Source: CAD feature listing. Evaluate the final solid. Frame: model axes, mm. A direction names the side the tool comes from. Round coordinates to 2 decimals unless told otherwise and drop trailing zeros. Order: outer loops, then holes, each group sorted by start corner. A loop starts at its lowest first (then second) coordinate and runs counter-clockwise, first axis right, second up. Notation, with made-up numbers: M 53,-7 L 66,-7 A14 cw 66,5 Z; hole C 20.25,48.25 d3. An arc over 180 degrees is marked long. Answer as CSV lines item,"result". Start each with the question number.
Item 1: Section query A-A on y = 9.75. Return the cut outline in (x, z).
Item 2: First-contact query: P1, Ø5.5, axis at x = 31, z = -31, coming from the +Y side; P2, Ø1.5, axis at x = 12.5, z = -29.5, coming from the +Y side. Flat tips, straight axial feed; report the tip coordinate or a pass-through.
Item 3: Set-up query: faces 4 (the face through (47.926, 8.378, -56.352)), 5 (the face through (12, 8.1, -30)), 6 (the face through (27, 6.4, -30)). Return all of +Z, -Z, +X, -X, +Y, -Y with unobstructed straight access to the full face (end or side cutting, diameter ignored); none if empty.
Item 4: Pull-direction query (Y, two-part tool) for faces 1 (the face through (9.62, 11, -30)), 2 (the face through (42.76, 15.983, -29.58)), 3 (the face through (4.14, 8.378, -56.983)); classes: +Y half, -Y half, draft (parallel to the pull), parting line (faces both ways), or undercut.
Item 5: Section query B-B on z = -5. State how many separate pieces and enclosed holes the cut face has, plus the area to 3 significant figures.
Item 6: Section query D-D on y = 3.5. Return the cut outline in (x, z), plus the area to 3 significant figures.
Item 7: Section query C-C on x = 49.4. Return the cut outline in (y, z) (3 decimals).
Item 8: Line query: line 1 (X direction, y = 7, z = -55); line 2 (X direction, y = 9, z = -24); line 3 (Z direction, x = 4.4, y = 4). Output: solid intervals per line, ascending. Write a range as [from, to].
from build123d import *

# Parameters (mm, degrees)
BOSS_EXTRUDE1_DEPTH             = 60
F_4_0MM_DOWEL_HOLE1_D           = 4
F_4_0MM_DOWEL_HOLE1_CSINK_D     = 4.05
F_4_0MM_DOWEL_HOLE1_CSINK_ANGLE = 90


with BuildPart() as part:
    # Sketch2 → Boss-Extrude1 (new body)
    with BuildSketch(Plane.XY):
        Polygon((36.38, 6.4), (26.9, 6.4), (26.9, 0), (53.8, 0), (53.8, 16.5), (44.18, 16.5), (41.3, 15.451765725), (41.3, 13.1), (44.18, 13.1), (44.18, 8.1), (39.18, 8.1), (39.18, 10.7), (36.38, 12.766601886), align=None)
    boss_extrude1 = extrude(amount=-BOSS_EXTRUDE1_DEPTH)

    # Mirror1: Boss-Extrude1 across plane
    add(boss_extrude1.mirror(Plane(origin=(26.9, 0, -60), x_dir=(0, 0, 1), z_dir=(1, 0, 0))))

    # Ø4.0mm Dowel Hole1 (through all)
    with Locations(Plane(origin=(0, 0, 0), x_dir=(-1, 0, 0), z_dir=(0, -1, 0))):
        with Locations((-49.4, 55), (-4.4, 55), (-4.4, 5), (-49.4, 5)):
            CounterSinkHole(F_4_0MM_DOWEL_HOLE1_D / 2, F_4_0MM_DOWEL_HOLE1_CSINK_D / 2, counter_sink_angle=F_4_0MM_DOWEL_HOLE1_CSINK_ANGLE)


solid = part.part
Results:
1,outline,"M 0,-60 L 9.62,-60 L 9.62,0 L 0,0 Z; M 14.62,-60 L 17.42,-60 L 17.42,0 L 14.62,0 Z; M 36.38,-60 L 39.18,-60 L 39.18,0 L 36.38,0 Z; M 44.18,-60 L 53.8,-60 L 53.8,0 L 44.18,0 Z; hole C 4.4,-55 d4; hole C 4.4,-5 d4; hole C 49.4,-55 d4; hole C 49.4,-5 d4"
2,P1,"y = 6.4"
2,P2,"y = 15.72"
3,face 4,"+Y, -Y"
3,face 5,"+Z, -Z"
3,face 6,"+Z, -Z, +Y"
4,face 1,"undercut"
4,face 2,"+Y half"
4,face 3,"draft"
5,separate pieces,"3"
5,enclosed holes,"0"
5,area,"470 mm^2"
6,outline,"M 0,-60 L 53.8,-60 L 53.8,0 L 0,0 Z; hole C 4.4,-55 d4; hole C 4.4,-5 d4; hole C 49.4,-55 d4; hole C 49.4,-5 d4"
6,area,"3,180 mm^2"
7,outline,"M 0,-60 L 16.5,-60 L 16.5,-57 L 0.025,-57 L 0,-57.025 Z; M 0,-52.975 L 0.025,-53 L 16.5,-53 L 16.5,-7 L 0.025,-7 L 0,-7.025 Z; M 0,-2.975 L 0.025,-3 L 16.5,-3 L 16.5,0 L 0,0 Z"
8,line 1,"[0, 2.4], [6.4, 17.42], [36.38, 47.4], [51.4, 53.8]"
8,line 2,"[0, 9.62], [14.62, 17.42], [36.38, 39.18], [44.18, 53.8]"
8,line 3,"[-60, -57], [-53, -7], [-3, 0]"
